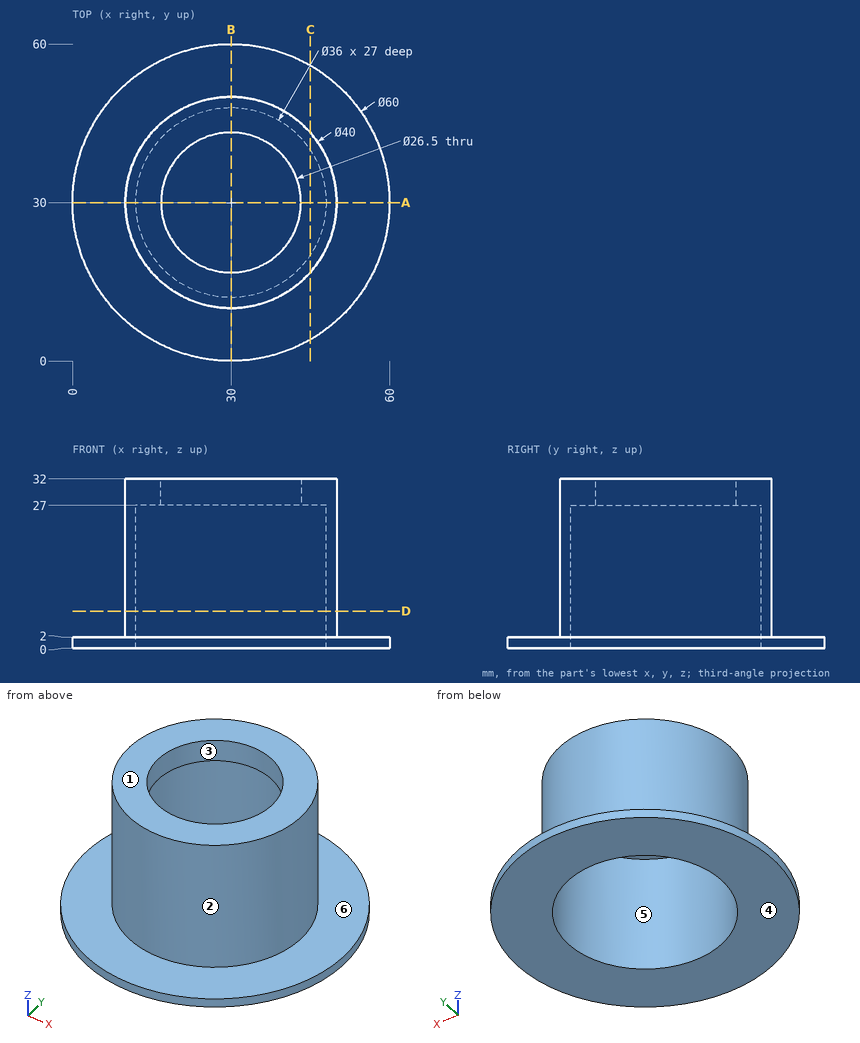
The drawing under review shows one solid part. Ordinate dimensions are in mm from its lowest x, y, z. A direction names the side the tool comes from. Coordinates: 2 decimals unless noted, no trailing zeros. Write each loop counter-clockwise with the first axis right and the second up, starting at its lowest first coordinate (ties: lowest second). Pieces come first, ordered by that corner, then holes. Notation, with made-up numbers: (6, 70.25) - (49, 70.25) arc R29 cw to (49, 93.25) - close; hole circle Ø5 at (18.25, 83.5). An arc over 180 degrees is marked (long way). Answer as CSV lines item,"result".
(1) Mouldability with a two-part tool opening along X and no side actions: class the marked faces 1, 2 and 3 as pulls with the +X half, pulls with the -X half, needs draft (parallel to the pull), parting line crosses it, or undercut.
Data:
face 1,"needs draft"
face 2,"parting line crosses it"
face 3,"undercut"
(2) Tool access review of the marked faces 4, 5 and 6: name each direction out of +Z, -Z, +X, -X, +Y, -Y from which nothing blocks a thin tool from reaching the whole face with its end or side.
Data:
face 4,"-Z, +X, -X, +Y, -Y"
face 5,"-Z"
face 6,"+Z"
(3) We need section C-C (x = 45). Give the boundary of the cut face in (y, z), plus the area to 3 significant figures.
Data:
outline,"(4.02, 0) - (20.05, 0) - (20.05, 27) - (39.95, 27) - (39.95, 0) - (55.98, 0) - (55.98, 2) - (43.23, 2) - (43.23, 32) - (16.77, 32) - (16.77, 2) - (4.02, 2) - close"
area,"360 mm2"
(4) We need section D-D (z = 7). Give the boundary of the cut face in (x, y), plus the area to 3 significant figures.
Data:
outline,"circle Ø40 at (30, 30); hole circle Ø36 at (30, 30)"
area,"239 mm2"
(5) We need section A-A (y = 30). Give the boundary of the cut face in (x, z).
Data:
outline,"(0, 0) - (12, 0) - (12, 27) - (16.75, 27) - (16.75, 32) - (10, 32) - (10, 2) - (0, 2) - close; (43.25, 27) - (48, 27) - (48, 0) - (60, 0) - (60, 2) - (50, 2) - (50, 32) - (43.25, 32) - close"
(6) For line 1 along X through (y, z) = (30, 7); line 2 along Y through (x, z) = (30, 30), list the stretches that pass through material, from the lowest coordinate up. Write a range as [from, to].
Data:
line 1,"x = [10, 12], [48, 50]"
line 2,"y = [10, 16.75], [43.25, 50]"
(7) Clearance check with flat-ended pins moving along their axes: pin 1 Ø6 at (y, z) = (47, 20) entering from +X; pin 2 Ø18 at (x, y) = (25.5, 26) entering from -Z; pin 3 Ø1 at (x, z) = (48.5, 16) entering from -Y. State where each tip first meets the part, or that it passes through.
Data:
pin 1,"stops at x = 44.28"
pin 2,"stops at z = 27"
pin 3,"stops at y = 21.28"
